For this review, take the finished solid that the model builds, in its own axes (mm). Face numbers are marked on the shaded views. Round coordinates to 2 decimals unless told otherwise and drop trailing zeros. Loops run counter-clockwise (first coordinate to the right, second up) from the corner with the lowest first, then second, coordinate; pieces in that order, holes last.
1) Mouldability with a two-part tool opening along X and no side actions: class the marked faces 1, 2, 3 and 4 as pulls with the +X half, pulls with the -X half, needs draft (parallel to the pull), parting line crosses it, or undercut.
2) Wall thickness on L1, parallel to Y at x = 10, z = 0.75; L2, parallel to X at y = -18, z = 1.3; L3, parallel to Y at x = 9, z = 0.9: over which ranges is each line inside the solid? List them lowest first.
3) Insertion check: pin 1 (0.9 mm diameter, centred on y = 2.5, z = 1.5, fed in from +X); pin 2 (6 mm diameter, centred on x = -10, y = -15.56, fed in from +Z); pin 3 (1.5 mm diameter, centred on x = -10, z = 1.5, fed in from +Y); pin 4 (1.5 mm diameter, centred on x = -17, y = 4.5, fed in from -Z). Each pin has a flat end and moves straight along its axis. Give the tip position at first contact, or say it passes through.
4) Take a section at B-B (y = 0). State the section outline as (x, z) points, then the cut area to 3 significant figures.
5) Take a section at A-A (x = 0). State the section outline as (y, z) points, then the cut area to 3 significant figures.
6) Take a section at C-C (z = 0.6). State the section outline as (x, y) points.
7) Take a section at D-D (y = -14). State the section outline as (x, z) points.
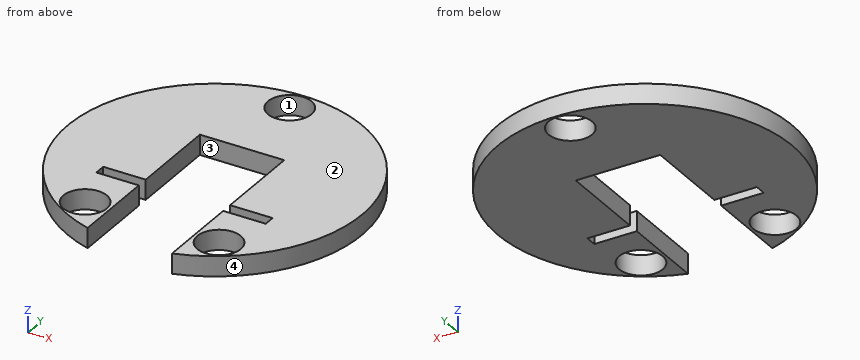
Autodesk Inventor part; units mm, degrees
ref_plane "Plan YZ" through (0, 0, 0) normal (1, 0, 0) x (0, 1, 0)
ref_plane "Plan XZ" through (0, 0, 0) normal (0, 1, 0) x (-1, 0, 0)
ref_plane "Plan XY" through (0, 0, 0) normal (0, 0, 1) x (1, 0, 0)
sketch "Esquisse1" plane through (0, 0, 0) normal (0, 0, 1) x (1, 0, 0)
  arc A0 (6.3, -21.0787) -> (-6.3, -21.0787) centre (0, 0) ccw
  line L0 (-6.3, 6.7) -> (6.3, 6.7)
  line L1 (-6.3, -6.7) -> (-12.65, -6.7)
  line L2 (-12.65, -8.4) -> (-12.65, -6.7)
  line L3 (-6.3, -8.4) -> (-12.65, -8.4)
  line L4 (6.3, -6.7) -> (12.65, -6.7)
  line L5 (12.65, -6.7) -> (12.65, -8.4)
  line L6 (12.65, -8.4) -> (6.3, -8.4)
  line L7 (-30.8, 0) -> (30.8, 0) construction
  line L8 (0, -29.7044) -> (0, 30.6757) construction
  line L9 (-6.3, -21.0787) -> (-6.3, -8.4)
  line L10 (-6.3, -6.7) -> (-6.3, 6.7)
  line L11 (6.3, -8.4) -> (6.3, -21.0787)
  line L12 (6.3, -21.0787) -> (6.3, -8.4) construction
  line L13 (6.3, -21.0787) -> (6.3, -8.4)
  line L14 (6.3, -6.7) -> (6.3, 6.7)
  dimension "d0" = 44
  dimension "d47" = 1.7
  dimension "d49" = 6.35
  dimension "d52" = 12.6
  dimension "d55" = 13.4
  dimension "d56" = 6.7
extrude "Extrusion1" add sketch "Esquisse1" along normal blind 3
sketch "Esquisse7" plane through (0, 0, 3) normal (0, 0, 1) x (1, 0, 0)
  circle A0 centre (0, 18.5) radius 3.25
  circle A1 centre (10, -15.5644) radius 3.25
  circle A2 centre (-10, -15.5644) radius 3.25
  line L0 (0, -29.6944) -> (0, 30.6157) construction
  circle A3 centre (0, 0) radius 18.5 construction
  dimension "d23" = 6.5
  dimension "d34" = 20
  dimension "d51" = 37
extrude "Extrusion5" cut sketch "Esquisse7" against normal through all
properties part number "S1702_couverclerailressort" material "Plastique PMMA"
Response:
1. face 1: undercut
1. face 2: needs draft
1. face 3: undercut
1. face 4: parting line crosses it
2. L1: y = -19.6 to -18.81, -12.31 to -8.4, -6.7 to 19.6
2. L2: x = -12.65 to -12.15, -7.85 to -6.3, 6.3 to 7.85, 12.15 to 12.65
2. L3: y = -20.07 to -18.66, -12.47 to -8.4, -6.7 to 20.07
3. pin 1: stops at x = 21.9
3. pin 2: passes through
3. pin 3: stops at y = 19.96
3. pin 4: stops at z = 0
4. outline: (-22, 0) - (-6.3, 0) - (-6.3, 3) - (-22, 3) - close; (6.3, 0) - (22, 0) - (22, 3) - (6.3, 3) - close
4. area: 94.2 mm2
5. outline: (6.7, 0) - (15.25, 0) - (15.25, 3) - (6.7, 3) - close; (21.75, 0) - (22, 0) - (22, 3) - (21.75, 3) - close
5. area: 26.4 mm2
6. outline: (-12.65, -8.4) - (-12.65, -6.7) - (-6.3, -6.7) - (-6.3, 6.7) - (6.3, 6.7) - (6.3, -6.7) - (12.65, -6.7) - (12.65, -8.4) - (6.3, -8.4) - (6.3, -21.08) arc R22 ccw (long way) to (-6.3, -21.08) - (-6.3, -8.4) - close; hole circle Ø6.5 at (-10, -15.56); hole circle Ø6.5 at (0, 18.5); hole circle Ø6.5 at (10, -15.56)
7. outline: (-16.97, 0) - (-12.85, 0) - (-12.85, 3) - (-16.97, 3) - close; (-7.15, 0) - (-6.3, 0) - (-6.3, 3) - (-7.15, 3) - close; (6.3, 0) - (7.15, 0) - (7.15, 3) - (6.3, 3) - close; (12.85, 0) - (16.97, 0) - (16.97, 3) - (12.85, 3) - close
